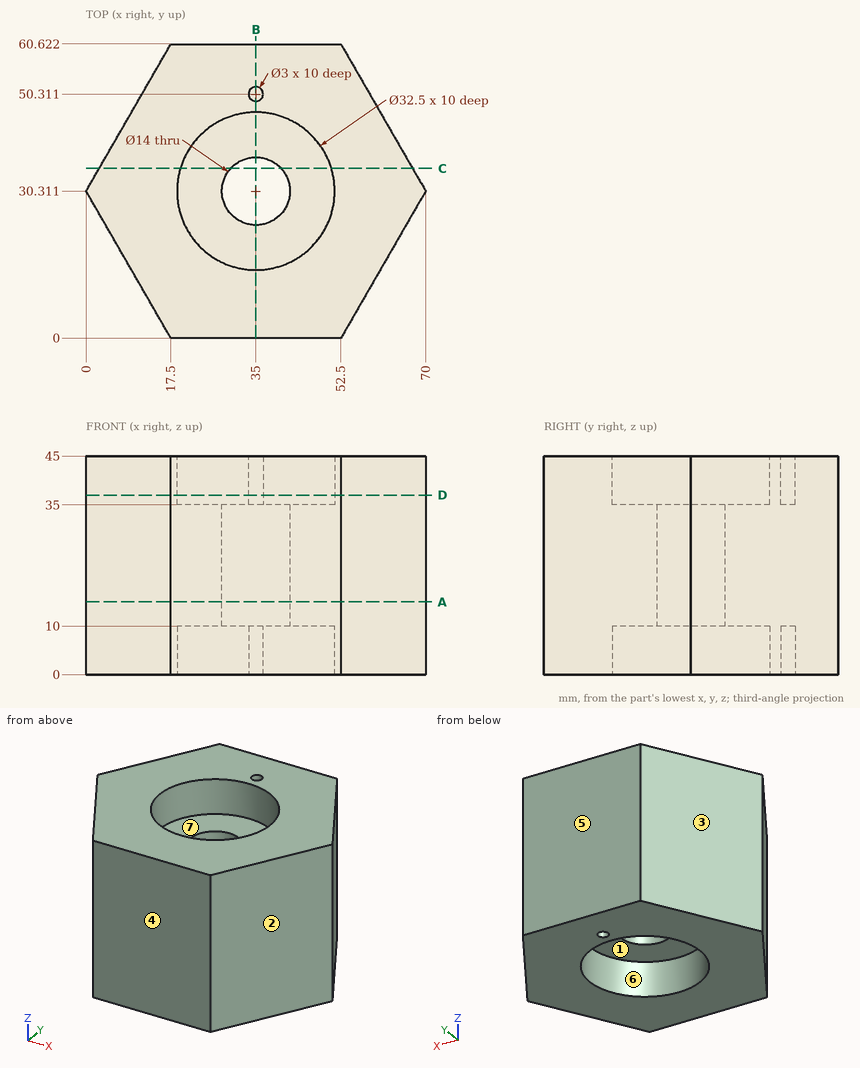
Geometry check sheet. Reference: drawing and pictorial views, mm from the part's lowest x, y, z. A direction names the side the tool comes from. Coordinates: 2 decimals unless noted, no trailing zeros. Order: outer loops, then holes, each group sorted by start corner. A loop starts at its lowest first (then second) coordinate and runs counter-clockwise, first axis right, second up. Notation, with made-up numbers: (-33, 89) - (-5, 89) arc R7 cw to (-5, 97) - close; hole circle Ø3 at (29.5, 6). An arc over 180 degrees is marked (long way). Answer in a Markdown table with one row per item. Add a question column.
1) Cross-section at B-B, the plane x = 35. Record the cut outline in (y, z).
2) Cross-section at A-A, the plane z = 15. Record the cut outline in (x, y).
3) Material ranges on line 1 along Y through (x, z) = (35, 3); line 2 along Y through (x, z) = (28.5, 6) (1 decimal); line 3 along Z through (x, y) = (45, 37), recorded low to high. Write a range as [from, to].
4) Gauge pin test, flat ends, axial feed: P1, Ø2.5, axis at x = 35, y = 50.31, coming from the -Z side; P2, Ø10, axis at x = 36, y = 27.5, coming from the +Z side; P3, Ø2, axis at y = 13, z = 29.5, coming from the +X side. Record the tip position at first contact, or that the pin passes through.
5) Cross-section at C-C, the plane y = 35. Record the cut outline in (x, z).
6) Set-up check for the marked faces 5, 6 and 7: record each of +Z, -Z, +X, -X, +Y, -Y from which the full face is reachable in a straight line by a thin tool's end or side.
7) Cross-section at D-D, the plane z = 37. Record the cut outline in (x, y).
8) Release check for a two-part mould opening along X. For the marked faces 1, 2, 3 and 4 record: +X half, -X half, draft (parallel to the pull), parting line (faces both ways), or undercut.
Check result:
| question | item | result |
|---|---|---|
| 1 | outline | (0, 0) - (14.06, 0) - (14.06, 10) - (23.31, 10) - (23.31, 35) - (14.06, 35) - (14.06, 45) - (0, 45) - close; (37.31, 10) - (46.56, 10) - (46.56, 0) - (48.81, 0) - (48.81, 10) - (51.81, 10) - (51.81, 0) - (60.62, 0) - (60.62, 45) - (51.81, 45) - (51.81, 35) - (48.81, 35) - (48.81, 45) - (46.56, 45) - (46.56, 35) - (37.31, 35) - close |
| 2 | outline | (0, 30.31) - (17.5, 0) - (52.5, 0) - (70, 30.31) - (52.5, 60.62) - (17.5, 60.62) - close; hole circle Ø14 at (35, 30.31) |
| 3 | line 1 | y = [0, 14.06], [46.56, 48.81], [51.81, 60.62] |
| 3 | line 2 | y = [0, 15.4], [45.2, 60.6] |
| 3 | line 3 | z = [10, 35] |
| 4 | P1 | stops at z = 10 |
| 4 | P2 | stops at z = 35 |
| 4 | P3 | stops at x = 60.58 |
| 5 | outline | (2.71, 0) - (19.44, 0) - (19.44, 10) - (29.8, 10) - (29.8, 35) - (19.44, 35) - (19.44, 45) - (2.71, 45) - close; (40.2, 10) - (50.56, 10) - (50.56, 0) - (67.29, 0) - (67.29, 45) - (50.56, 45) - (50.56, 35) - (40.2, 35) - close |
| 6 | face 5 | +Z, -Z, +X, -X, +Y |
| 6 | face 6 | -Z |
| 6 | face 7 | +Z |
| 7 | outline | (0, 30.31) - (17.5, 0) - (52.5, 0) - (70, 30.31) - (52.5, 60.62) - (17.5, 60.62) - close; hole circle Ø32.5 at (35, 30.31); hole circle Ø3 at (35, 50.31) |
| 8 | face 1 | undercut |
| 8 | face 2 | +X half |
| 8 | face 3 | -X half |
| 8 | face 4 | draft |
